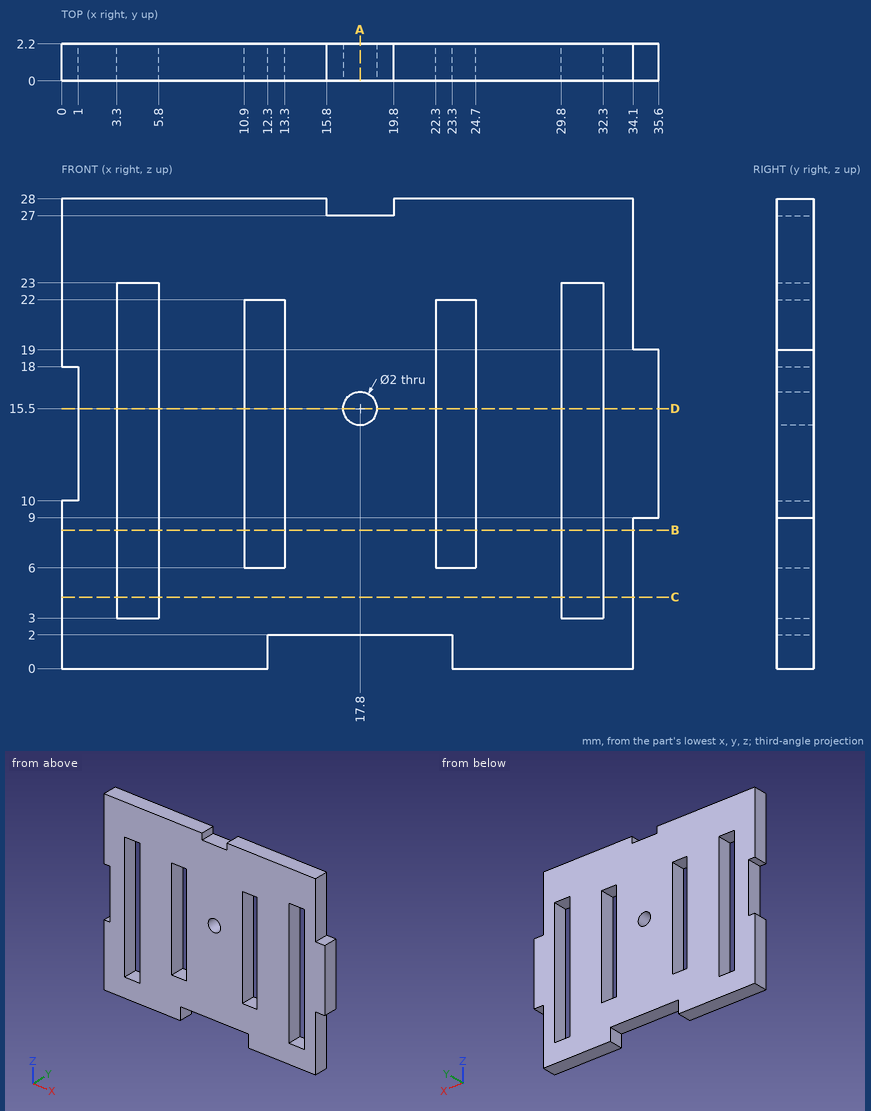
Drawing for the job (mm, zero at the part's lowest x, y, z). Give positions to 0.01 mm unless a question says otherwise; leave off trailing zeros. Order: outer loops, then holes, each group sorted by start corner. A loop starts at its lowest first (then second) coordinate and runs counter-clockwise, first axis right, second up. Notation, with made-up numbers: M -17.5,31 L -11.5,31 A36 ccw -11.5,66 Z; hole C 34.25,49.5 d3. An arc over 180 degrees is marked long. Use a Markdown table: item, result. Add a question column.
(1) Probe line 1 along X through (y, z) = (0.3, 8); line 2 along X through (y, z) = (1, 15.5); line 3 along X through (y, z) = (0.2, 14). List the from-to ranges inside material, lowest first. Write a range as [from, to].
(2) Drop flat-ended pins along their axis: P1, Ø1.1, axis at y = 1.5, z = 27.5, coming from the +X side; P2, Ø1.1, axis at y = 1.5, z = 14.5, coming from the -X side; P3, Ø0.8, axis at x = 35, y = 1, coming from the -Z side. Give the stop position or say it passes through.
(3) Saw through at C-C, the plane z = 4.25. Give the cut face in (x, y), and give its area (3 significant figures).
(4) Saw through at B-B, the plane z = 8.25. Give the cut face in (x, y), and give its area (3 significant figures).
(5) Saw through at A-A, the plane x = 17.8. Give the cut face in (y, z).
(6) Saw through at D-D, the plane z = 15.5. Give the cut face in (x, y), and give its area (3 significant figures).
Answer key:
| question | item | result |
|---|---|---|
| 1 | line 1 | [0, 3.3], [5.8, 10.9], [13.3, 22.3], [24.7, 29.8], [32.3, 34.1] |
| 1 | line 2 | [1, 3.3], [5.8, 10.9], [13.3, 16.8], [18.8, 22.3], [24.7, 29.8], [32.3, 35.6] |
| 1 | line 3 | [1, 3.3], [5.8, 10.9], [13.3, 22.3], [24.7, 29.8], [32.3, 35.6] |
| 2 | P1 | x = 34.1 |
| 2 | P2 | x = 1 |
| 2 | P3 | z = 9 |
| 3 | outline | M 0,0 L 3.3,0 L 3.3,2.2 L 0,2.2 Z; M 5.8,0 L 29.8,0 L 29.8,2.2 L 5.8,2.2 Z; M 32.3,0 L 34.1,0 L 34.1,2.2 L 32.3,2.2 Z |
| 3 | area | 64.0 mm^2 |
| 4 | outline | M 0,0 L 3.3,0 L 3.3,2.2 L 0,2.2 Z; M 5.8,0 L 10.9,0 L 10.9,2.2 L 5.8,2.2 Z; M 13.3,0 L 22.3,0 L 22.3,2.2 L 13.3,2.2 Z; M 24.7,0 L 29.8,0 L 29.8,2.2 L 24.7,2.2 Z; M 32.3,0 L 34.1,0 L 34.1,2.2 L 32.3,2.2 Z |
| 4 | area | 53.5 mm^2 |
| 5 | outline | M 0,2 L 2.2,2 L 2.2,14.5 L 0,14.5 Z; M 0,16.5 L 2.2,16.5 L 2.2,27 L 0,27 Z |
| 6 | outline | M 1,0 L 3.3,0 L 3.3,2.2 L 1,2.2 Z; M 5.8,0 L 10.9,0 L 10.9,2.2 L 5.8,2.2 Z; M 13.3,0 L 16.8,0 L 16.8,2.2 L 13.3,2.2 Z; M 18.8,0 L 22.3,0 L 22.3,2.2 L 18.8,2.2 Z; M 24.7,0 L 29.8,0 L 29.8,2.2 L 24.7,2.2 Z; M 32.3,0 L 35.6,0 L 35.6,2.2 L 32.3,2.2 Z |
| 6 | area | 50.2 mm^2 |
